```python
from build123d import *

# Parameters (mm, degrees)
SKETCH4_R           = 17
BOSS_EXTRUDE2_DEPTH = 3
SKETCH5_R           = 7
BOSS_EXTRUDE3_DEPTH = 1.5
CUT_EXTRUDE2_DEPTH  = 25.459149617
CUT_EXTRUDE3_DEPTH  = 25.228082879


with BuildPart() as part:
    # Sketch4 → Boss-Extrude2 (new body)
    with BuildSketch(Plane.XY):
        Circle(SKETCH4_R)
    extrude(amount=BOSS_EXTRUDE2_DEPTH)

    # Sketch5 → Boss-Extrude3 (add)
    with BuildSketch(Plane.XY.offset(3)):
        Circle(SKETCH5_R)
    extrude(amount=BOSS_EXTRUDE3_DEPTH)

    # Sketch3 → Cut-Extrude2 (cut, through all)
    with BuildSketch(Plane(origin=(0, 0, 0), x_dir=(-1, 0, 0), z_dir=(0, 0, 1))):
        with BuildLine():
            Line((-2.185, 1.975), (2.185, 1.975))
            ThreePointArc((2.185, 1.975), (2.931974702, 0), (2.185, -1.975))
            Line((2.185, -1.975), (-2.185, -1.975))
            ThreePointArc((-2.185, -1.975), (-2.931974702, 0), (-2.185, 1.975))
        make_face()
    extrude(amount=CUT_EXTRUDE2_DEPTH, mode=Mode.SUBTRACT)

    # Sketch6 → Cut-Extrude3 (cut, through all)
    with BuildSketch(Plane.XY.offset(3)):
        with BuildLine():
            Line((11, 0.914805145), (15, 0.914805145))
            ThreePointArc((15, 0.914805145), (15.914805145, 0), (15, -0.914805145))
            Line((15, -0.914805145), (11, -0.914805145))
            ThreePointArc((11, -0.914805145), (10.085194855, 0), (11, 0.914805145))
        make_face()
        with BuildLine():
            Line((10.744312015, -2.529155544), (14.548538081, -3.765223522))
            ThreePointArc((14.548538081, -3.765223522), (15.135879138, -4.917945252), (13.983157408, -5.50528631))
            Line((13.983157408, -5.50528631), (10.178931343, -4.269218332))
            ThreePointArc((10.178931343, -4.269218332), (9.591590285, -3.116496602), (10.744312015, -2.529155544))
        make_face()
        with BuildLine():
            Line((9.436895911, -5.725544867), (12.672963888, -8.076685876))
            ThreePointArc((12.672963888, -8.076685876), (12.875347824, -9.354487757), (11.597545943, -9.556871693))
            Line((11.597545943, -9.556871693), (8.361477965, -7.205730684))
            ThreePointArc((8.361477965, -7.205730684), (8.15909403, -5.927928803), (9.436895911, -5.725544867))
        make_face()
        with BuildLine():
            Line((7.205730684, -8.361477965), (9.556871693, -11.597545943))
            ThreePointArc((9.556871693, -11.597545943), (9.354487757, -12.875347824), (8.076685876, -12.672963888))
            Line((8.076685876, -12.672963888), (5.725544867, -9.436895911))
            ThreePointArc((5.725544867, -9.436895911), (5.927928803, -8.15909403), (7.205730684, -8.361477965))
        make_face()
        with BuildLine():
            Line((4.269218332, -10.178931343), (5.50528631, -13.983157408))
            ThreePointArc((5.50528631, -13.983157408), (4.917945252, -15.135879138), (3.765223522, -14.548538081))
            Line((3.765223522, -14.548538081), (2.529155544, -10.744312015))
            ThreePointArc((2.529155544, -10.744312015), (3.116496602, -9.591590285), (4.269218332, -10.178931343))
        make_face()
        with BuildLine():
            Line((0.914805145, -11), (0.914805145, -15))
            ThreePointArc((0.914805145, -15), (0, -15.914805145), (-0.914805145, -15))
            Line((-0.914805145, -15), (-0.914805145, -11))
            ThreePointArc((-0.914805145, -11), (0, -10.085194855), (0.914805145, -11))
        make_face()
        with BuildLine():
            Line((-2.529155544, -10.744312015), (-3.765223522, -14.548538081))
            ThreePointArc((-3.765223522, -14.548538081), (-4.917945252, -15.135879138), (-5.50528631, -13.983157408))
            Line((-5.50528631, -13.983157408), (-4.269218332, -10.178931343))
            ThreePointArc((-4.269218332, -10.178931343), (-3.116496602, -9.591590285), (-2.529155544, -10.744312015))
        make_face()
        with BuildLine():
            Line((-5.725544867, -9.436895911), (-8.076685876, -12.672963888))
            ThreePointArc((-8.076685876, -12.672963888), (-9.354487757, -12.875347824), (-9.556871693, -11.597545943))
            Line((-9.556871693, -11.597545943), (-7.205730684, -8.361477965))
            ThreePointArc((-7.205730684, -8.361477965), (-5.927928803, -8.15909403), (-5.725544867, -9.436895911))
        make_face()
        with BuildLine():
            Line((-8.361477965, -7.205730684), (-11.597545943, -9.556871693))
            ThreePointArc((-11.597545943, -9.556871693), (-12.875347824, -9.354487757), (-12.672963888, -8.076685876))
            Line((-12.672963888, -8.076685876), (-9.436895911, -5.725544867))
            ThreePointArc((-9.436895911, -5.725544867), (-8.15909403, -5.927928803), (-8.361477965, -7.205730684))
        make_face()
        with BuildLine():
            Line((-10.178931343, -4.269218332), (-13.983157408, -5.50528631))
            ThreePointArc((-13.983157408, -5.50528631), (-15.135879138, -4.917945252), (-14.548538081, -3.765223522))
            Line((-14.548538081, -3.765223522), (-10.744312015, -2.529155544))
            ThreePointArc((-10.744312015, -2.529155544), (-9.591590285, -3.116496602), (-10.178931343, -4.269218332))
        make_face()
        with BuildLine():
            Line((-11, -0.914805145), (-15, -0.914805145))
            ThreePointArc((-15, -0.914805145), (-15.914805145, 0), (-15, 0.914805145))
            Line((-15, 0.914805145), (-11, 0.914805145))
            ThreePointArc((-11, 0.914805145), (-10.085194855, 0), (-11, -0.914805145))
        make_face()
        with BuildLine():
            Line((-10.744312015, 2.529155544), (-14.548538081, 3.765223522))
            ThreePointArc((-14.548538081, 3.765223522), (-15.135879138, 4.917945252), (-13.983157408, 5.50528631))
            Line((-13.983157408, 5.50528631), (-10.178931343, 4.269218332))
            ThreePointArc((-10.178931343, 4.269218332), (-9.591590285, 3.116496602), (-10.744312015, 2.529155544))
        make_face()
        with BuildLine():
            Line((-9.436895911, 5.725544867), (-12.672963888, 8.076685876))
            ThreePointArc((-12.672963888, 8.076685876), (-12.875347824, 9.354487757), (-11.597545943, 9.556871693))
            Line((-11.597545943, 9.556871693), (-8.361477965, 7.205730684))
            ThreePointArc((-8.361477965, 7.205730684), (-8.15909403, 5.927928803), (-9.436895911, 5.725544867))
        make_face()
        with BuildLine():
            Line((-7.205730684, 8.361477965), (-9.556871693, 11.597545943))
            ThreePointArc((-9.556871693, 11.597545943), (-9.354487757, 12.875347824), (-8.076685876, 12.672963888))
            Line((-8.076685876, 12.672963888), (-5.725544867, 9.436895911))
            ThreePointArc((-5.725544867, 9.436895911), (-5.927928803, 8.15909403), (-7.205730684, 8.361477965))
        make_face()
        with BuildLine():
            Line((-4.269218332, 10.178931343), (-5.50528631, 13.983157408))
            ThreePointArc((-5.50528631, 13.983157408), (-4.917945252, 15.135879138), (-3.765223522, 14.548538081))
            Line((-3.765223522, 14.548538081), (-2.529155544, 10.744312015))
            ThreePointArc((-2.529155544, 10.744312015), (-3.116496602, 9.591590285), (-4.269218332, 10.178931343))
        make_face()
        with BuildLine():
            Line((-0.914805145, 11), (-0.914805145, 15))
            ThreePointArc((-0.914805145, 15), (0, 15.914805145), (0.914805145, 15))
            Line((0.914805145, 15), (0.914805145, 11))
            ThreePointArc((0.914805145, 11), (0, 10.085194855), (-0.914805145, 11))
        make_face()
        with BuildLine():
            Line((2.529155544, 10.744312015), (3.765223522, 14.548538081))
            ThreePointArc((3.765223522, 14.548538081), (4.917945252, 15.135879138), (5.50528631, 13.983157408))
            Line((5.50528631, 13.983157408), (4.269218332, 10.178931343))
            ThreePointArc((4.269218332, 10.178931343), (3.116496602, 9.591590285), (2.529155544, 10.744312015))
        make_face()
        with BuildLine():
            Line((5.725544867, 9.436895911), (8.076685876, 12.672963888))
            ThreePointArc((8.076685876, 12.672963888), (9.354487757, 12.875347824), (9.556871693, 11.597545943))
            Line((9.556871693, 11.597545943), (7.205730684, 8.361477965))
            ThreePointArc((7.205730684, 8.361477965), (5.927928803, 8.15909403), (5.725544867, 9.436895911))
        make_face()
        with BuildLine():
            Line((8.361477965, 7.205730684), (11.597545943, 9.556871693))
            ThreePointArc((11.597545943, 9.556871693), (12.875347824, 9.354487757), (12.672963888, 8.076685876))
            Line((12.672963888, 8.076685876), (9.436895911, 5.725544867))
            ThreePointArc((9.436895911, 5.725544867), (8.15909403, 5.927928803), (8.361477965, 7.205730684))
        make_face()
        with BuildLine():
            Line((10.178931343, 4.269218332), (13.983157408, 5.50528631))
            ThreePointArc((13.983157408, 5.50528631), (15.135879138, 4.917945252), (14.548538081, 3.765223522))
            Line((14.548538081, 3.765223522), (10.744312015, 2.529155544))
            ThreePointArc((10.744312015, 2.529155544), (9.591590285, 3.116496602), (10.178931343, 4.269218332))
        make_face()
    extrude(amount=-CUT_EXTRUDE3_DEPTH, mode=Mode.SUBTRACT)


solid = part.part
```
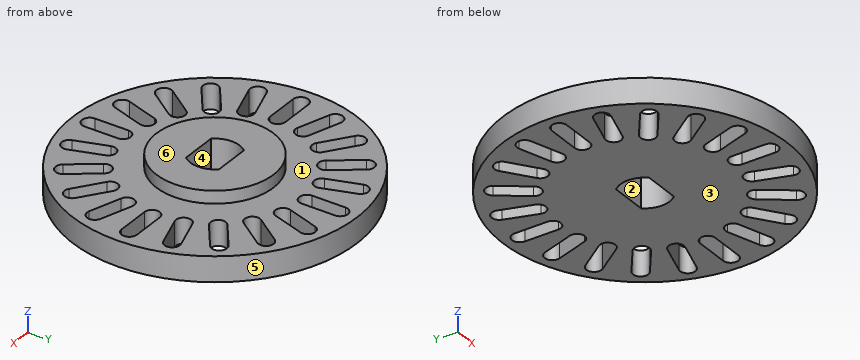
Read the model definition and answer for the solid it produces. Units are mm, in the model's axes. Face numbers are marked on the shaded views. A direction names the side the tool comes from. Give positions to 0.01 mm unless a question says otherwise; leave off trailing zeros. Write each loop counter-clockwise with the first axis right and the second up, starting at its lowest first coordinate (ties: lowest second). Pieces come first, ordered by that corner, then holes. Notation, with made-up numbers: M 58.5,66 L 68.5,66 A20 cw 68.5,96 Z; hole C 21.25,47.25 d8. An arc over 180 degrees is marked long. Put each result on its own line as item: value. Start each with the question number.
1. Consider line 1 along X through (y, z) = (15, 2.6); line 2 along Y through (x, z) = (11.5, 1.55); line 3 along Y through (x, z) = (7, 2.6). Determine where each line is inside the solid, lowest interval first.
2. The part is cut by section D-D, the plane z = 1.7. Give the number of separate pieces and of enclosed holes in the cut face, and give its area (3 significant figures).
3. The part is cut by section A-A, the plane x = 0. Give the vertices of the cut face in (y, z) (3 decimals).
4. The part is cut by section C-C, the plane x = -5. Give the vertices of the cut face in (y, z), and give its area (3 significant figures).
5. The part is cut by section B-B, the plane z = 3.7. Give the vertices of the cut face in (x, y) (3 decimals).
6. Which of the six approach directions +Z, -Z, +X, -X, +Y, -Y give full straight-line access (tool end or side, diameter ignored) to the marked faces 1, 2 and 3?
7. For a pull along Y with two mould halves and no side action, classify the marked faces 4, 5 and 6 as released by +Y, released by -Y, zero draft, split by the parting line, or undercut.
8. Each of these flat-tipped pins is pushed along its axis until it touches: pin 1 Ø1.5 at (x, z) = (-12, 2) entering from -Y; pin 2 Ø0.9 at (y, z) = (13, 1) entering from +X; pin 3 Ø1.5 at (x, z) = (13, 1.5) entering from +Y. Where does it stop, or does it pass through?
Final values:
1. line 1: x = -8 to -5.18, -4.09 to -0.91, 0.91 to 4.09, 5.18 to 8
1. line 2: y = -12.52 to -9.49, -7.22 to -4.7, -2.77 to -0.91, 0.91 to 2.77, 4.7 to 7.22, 9.49 to 12.52
1. line 3: y = -15.49 to -11.19, -8.16 to 8.16, 11.19 to 15.49
2. separate pieces: 1
2. enclosed holes: 21
2. area: 688 mm²
3. outline: M -17,0 L -15.915,0 L -15.915,3 L -17,3 Z; M -10.085,0 L -1.975,0 L -1.975,4.5 L -7,4.5 L -7,3 L -10.085,3 Z; M 1.975,0 L 10.085,0 L 10.085,3 L 7,3 L 7,4.5 L 1.975,4.5 Z; M 15.915,0 L 17,0 L 17,3 L 15.915,3 Z
4. outline: M -16.25,0 L -15.1,0 L -15.1,3 L -16.25,3 Z; M -12.43,0 L 12.43,0 L 12.43,3 L 4.9,3 L 4.9,4.5 L -4.9,4.5 L -4.9,3 L -12.43,3 Z; M 15.1,0 L 16.25,0 L 16.25,3 L 15.1,3 Z
4. area: 96.1 mm²
5. outline: C 0,0 d14; hole M -2.185,-1.975 L 2.185,-1.975 A2.984 ccw 2.185,1.975 L -2.185,1.975 A2.984 ccw Z
6. face 1: +Z
6. face 2: +Z, -Z
6. face 3: -Z, +X, -X, +Y, -Y
7. face 4: undercut
7. face 5: split by the parting line
7. face 6: zero draft
8. pin 1: stops at y = -12.75
8. pin 2: stops at x = 11.47
8. pin 3: stops at y = 11.79
